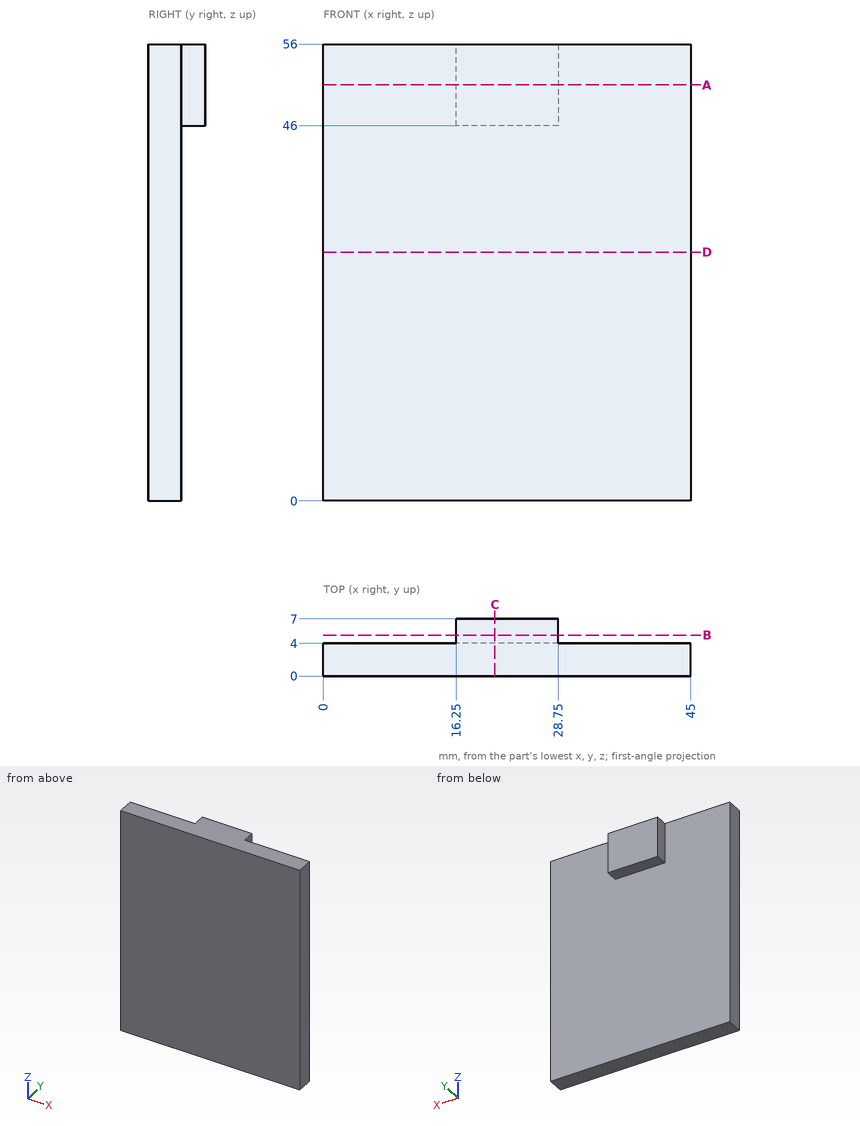
Drawing for the job (mm, zero at the part's lowest x, y, z). Round coordinates to 2 decimals unless told otherwise and drop trailing zeros. Loops run counter-clockwise (first coordinate to the right, second up) from the corner with the lowest first, then second, coordinate; pieces in that order, holes last.
1. Band-saw the part on A-A, the plane z = 51. List the corners of the cut face in (x, y), and give its area (4 significant figures).
Check values:
outline: (0, 0) - (45, 0) - (45, 4) - (28.75, 4) - (28.75, 7) - (16.25, 7) - (16.25, 4) - (0, 4) - close
area: 217.5 mm2
2. Band-saw the part on C-C, the plane x = 21. List the corners of the cut face in (y, z), and give its area (3 significant figures).
Check values:
outline: (0, 0) - (4, 0) - (4, 46) - (7, 46) - (7, 56) - (0, 56) - close
area: 254 mm2
3. Band-saw the part on B-B, the plane y = 5. List the corners of the cut face in (x, z), and give its area (3 significant figures).
Check values:
outline: (16.25, 46) - (28.75, 46) - (28.75, 56) - (16.25, 56) - close
area: 125 mm2
4. Band-saw the part on D-D, the plane z = 30.5. List the corners of the cut face in (x, y).
Check values:
outline: (0, 0) - (45, 0) - (45, 4) - (0, 4) - close
5. Drop flat-ended pins along their axis: P1, Ø2.5, axis at x = 24, y = 5.5, coming from the -Z side; P2, Ø0.9, axis at y = 5, z = 53, coming from the -X side; P3, Ø0.9, axis at y = 6, z = 50.5, coming from the +X side. Give the stop position or say it passes through.
Check values:
P1: stops at z = 46
P2: stops at x = 16.25
P3: stops at x = 28.75
6. Wall check: probe 1 along Y at (x, z) = (21, 23.5); probe 2 along Z at (x, y) = (26.5, 6.75). Give the ranges that are in metal, low to high.
Check values:
probe 1: y = 0 to 4
probe 2: z = 46 to 56
